CAD build for the part. Positions are in the model's coordinates, mm. Face numbers are marked on the shaded views. A direction names the side the tool comes from. Give positions to 0.01 mm unless a question says otherwise; leave off trailing zeros. Loops run counter-clockwise (first coordinate to the right, second up) from the corner with the lowest first, then second, coordinate; pieces in that order, holes last.
```python
from build123d import *

# Parameters (mm, degrees)
F0_R     = 49.9731951159
F1_DEPTH = 30
F2_R     = 22.7581218929
F3_DEPTH = 60
F4_T     = -3


with BuildPart() as f1:
    # F0 (on Top) → F1 (new body)
    with BuildSketch(Plane.XY):
        Circle(F0_R)
    extrude(amount=-F1_DEPTH)

    # F2 (on face) → F3 (join)
    with BuildSketch(Plane.XY):
        with Locations((-13.4756937623, -21.6836426407)):
            Circle(F2_R)
    extrude(amount=F3_DEPTH)

    # F4 (hollow: no face is removed)
    offset(amount=F4_T, kind=Kind.INTERSECTION, mode=Mode.SUBTRACT)


solid = f1.part
```
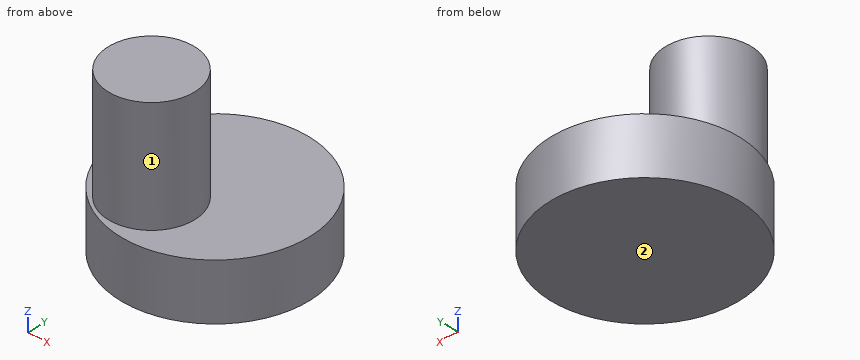
1. Tool access for the marked faces 1 and 2: list every direction of +Z, -Z, +X, -X, +Y, -Y with a clear straight run to the whole face (end or side of a thin tool).
Responses:
face 1: +Z
face 2: -Z, +X, -X, +Y, -Y
2. Drop flat-ended pins along their axis: pin 1 (10 mm diameter, centred on x = -39, z = -9.5, fed in from +Y); pin 2 (3 mm diameter, centred on x = -28, z = 17, fed in from -Y); pin 3 (1 mm diameter, centred on y = -19.5, z = -7.5, fed in from -X). Give the stop position or say it passes through.
Responses:
pin 1: stops at y = 36.62
pin 2: stops at y = -40.35
pin 3: stops at x = -46.22
3. Saw through at A-A, the plane y = -35. List the corners of the cut face in (x, z).
Responses:
outline: (-35.67, -30) - (35.67, -30) - (35.67, 0) - (4.98, 0) - (4.98, 60) - (-31.93, 60) - (-31.93, 0) - (-35.67, 0) - close; hole (-31.33, -27) - (31.33, -27) - (31.33, -3) - (1.12, -3) - (1.12, 57) - (-28.07, 57) - (-28.07, -3) - (-31.33, -3) - close
4. Probe line 1 along Y through (x, z) = (-1.5, -22); line 2 along X through (y, z) = (-21, 43); line 3 along Z through (x, y) = (-35, 16). List the from-to ranges inside material, lowest first.
Responses:
line 1: y = -49.95 to -46.95, 46.95 to 49.95
line 2: x = -36.22 to -33.22, 6.27 to 9.27
line 3: z = -30 to -27, -3 to 0
5. Saw through at D-D, the plane x = 43. List the corners of the cut face in (y, z), and give its area (3 significant figures).
Responses:
outline: (-25.46, -30) - (25.46, -30) - (25.46, 0) - (-25.46, 0) - close; hole (-18.91, -27) - (18.91, -27) - (18.91, -3) - (-18.91, -3) - close
area: 620 mm2
6. Saw through at B-B, the plane x = -0.5. List the corners of the cut face in (y, z), and give its area (3 significant figures).
Responses:
outline: (-49.97, -30) - (49.97, -30) - (49.97, 0) - (-2.99, 0) - (-2.99, 60) - (-40.38, 60) - (-40.38, 0) - (-49.97, 0) - close; hole (-46.97, -27) - (46.97, -27) - (46.97, -3) - (-6.78, -3) - (-6.78, 57) - (-36.58, 57) - (-36.58, -3) - (-46.97, -3) - close
area: 1,200 mm2
7. Saw through at C-C, the plane z = -12. List the corners of the cut face in (x, y).
Responses:
outline: circle Ø99.95 at (0, 0); hole circle Ø93.95 at (0, 0)
